```python
from build123d import *

# Parameters (mm, degrees)
SKETCH1_R           = 1
SKETCH1_R_2         = 5.5
BOSS_EXTRUDE1_DEPTH = 3


with BuildPart() as part:
    # Sketch1 → Boss-Extrude1 (new body)
    with BuildSketch(Plane.XY):
        with BuildLine():
            Line((0, 20), (70, 20))
            ThreePointArc((70, 20), (90, 0), (70, -20))
            Line((70, -20), (0, -20))
            ThreePointArc((0, -20), (-20, 0), (0, 20))
        make_face()
        with Locations((10, 0)):
            Circle(SKETCH1_R, mode=Mode.SUBTRACT)
        with Locations((0, -10)):
            Circle(SKETCH1_R, mode=Mode.SUBTRACT)
        with Locations((-10, 0)):
            Circle(SKETCH1_R, mode=Mode.SUBTRACT)
        with Locations((0, 10)):
            Circle(SKETCH1_R, mode=Mode.SUBTRACT)
        with Locations((80, 0)):
            Circle(SKETCH1_R, mode=Mode.SUBTRACT)
        with Locations((60, 0)):
            Circle(SKETCH1_R, mode=Mode.SUBTRACT)
        with Locations((70, 10)):
            Circle(SKETCH1_R, mode=Mode.SUBTRACT)
        with Locations((70, -10)):
            Circle(SKETCH1_R, mode=Mode.SUBTRACT)
        Circle(SKETCH1_R_2, mode=Mode.SUBTRACT)
        with Locations((70, 0)):
            Circle(SKETCH1_R_2, mode=Mode.SUBTRACT)
    extrude(amount=BOSS_EXTRUDE1_DEPTH)


solid = part.part
```
Geometry check sheet. Reference: the model listing, model coordinates, mm. Coordinates: 2 decimals unless noted, no trailing zeros. Order: outer loops, then holes, each group sorted by start corner. A loop starts at its lowest first (then second) coordinate and runs counter-clockwise, first axis right, second up.
Item 1: Section check A-A (y = 0). Enter the section's corners in (x, z), plus the area to 3 significant figures.
Item 2: Section check B-B (z = 0.6). Count the separate pieces of the cut face and the enclosed holes in it, plus the area to 3 significant figures.
Item 3: Section check C-C (y = 10). Enter the section's corners in (x, z), plus the area to 3 significant figures.
Item 4: Mould release check, pull along X, two halves, no side actions. Record for faces 1 (the flat face through (36, 0, 3)), 2 (the cylindrical face through (-1.19, -5.37, 1.48)), 3 (the cylindrical face through (90, 0, 1)), 4 (the cylindrical face through (64.505, 0.242, 1.479)): released by +X, released by -X, zero draft, split by the parting line, or undercut.
Item 5: Depth check by flat-ended pin: pin 1 (14.5 mm diameter, centred on x = 70, y = 0, fed in from -Z). Enter the tip coordinate at first touch or a pass-through.
Item 6: Section check D-D (x = -10). Enter the section's corners in (y, z), plus the area to 3 significant figures.
Item 7: Scan lines: line 1 along Y through (x, z) = (70, 1.45); line 2 along Y through (x, z) = (60, 1.05); line 3 along X through (y, z) = (3, 1.9). Record each from-to range of solid material in increasing order.
Check sheet entries:
1. outline: (-20, 0) - (-11, 0) - (-11, 3) - (-20, 3) - close; (-9, 0) - (-5.5, 0) - (-5.5, 3) - (-9, 3) - close; (5.5, 0) - (9, 0) - (9, 3) - (5.5, 3) - close; (11, 0) - (59, 0) - (59, 3) - (11, 3) - close; (61, 0) - (64.5, 0) - (64.5, 3) - (61, 3) - close; (75.5, 0) - (79, 0) - (79, 3) - (75.5, 3) - close; (81, 0) - (90, 0) - (90, 3) - (81, 3) - close
1. area: 240 mm2
2. separate pieces: 1
2. enclosed holes: 10
2. area: 3,840 mm2
3. outline: (-17.32, 0) - (-1, 0) - (-1, 3) - (-17.32, 3) - close; (1, 0) - (69, 0) - (69, 3) - (1, 3) - close; (71, 0) - (87.32, 0) - (87.32, 3) - (71, 3) - close
3. area: 302 mm2
4. face 1: zero draft
4. face 2: undercut
4. face 3: released by +X
4. face 4: undercut
5. pin 1: stops at z = 0
6. outline: (-17.32, 0) - (-1, 0) - (-1, 3) - (-17.32, 3) - close; (1, 0) - (17.32, 0) - (17.32, 3) - (1, 3) - close
6. area: 97.9 mm2
7. line 1: y = -20 to -11, -9 to -5.5, 5.5 to 9, 11 to 20
7. line 2: y = -20 to -1, 1 to 20
7. line 3: x = -19.77 to -4.61, 4.61 to 65.39, 74.61 to 89.77
